Can you work these out from the model? Positions are in its coordinate system, mm. A direction names the side the tool comes from. Round coordinates to 2 decimals unless told otherwise and drop trailing zeros. Write each loop counter-clockwise with the first axis right and the second up, starting at its lowest first coordinate (ties: lowest second). Pieces come first, ordered by that corner, then holes. Notation, with made-up numbers: M 18,1 L 74,1 A29 cw 74,22 Z; hole C 87.5,-17.75 d3. An arc over 180 degrees is marked long. Answer in a Markdown table with one row per item. Add a question column.
(1) For faces 4 (the face through (48, 3, 2)), 5 (the face through (35.1, 3, -10)), 6 (the face through (81, 3, 2)), 7 (the face through (5, 3, 2)), 8 (the face through (2, 3, -8)), which set-ups out of +Z, -Z, +X, -X, +Y, -Y let a thin tool reach every point of the face, with its end or its side?
(2) Suppose I cut it at C-C, the plane x = 45. Write out the boundary of the cut face in (y, z), then the cut area to 3 significant figures.
(3) Suppose I cut it at B-B, the plane z = -11.5. Write out the boundary of the cut face in (x, y).
(4) If we mould it in two halves opening along X, with no side actions, what happens to faces 1 (the face through (59, 3, 0)), 2 (the face through (78.8, 3, -10)), 3 (the face through (42, 6, -4))? For each: released by +X, released by -X, zero draft, split by the parting line, or undercut.
(5) I'm going to push flat-ended pins straight in: pin 1 (1.5 mm diameter, centred on x = 83.5, y = 2, fed in from +Z); pin 2 (1.8 mm diameter, centred on x = 83.5, y = 4, fed in from -Z); pin 3 (1.5 mm diameter, centred on y = 2, z = -11, fed in from +X). Where does each tip first touch, or does it pass through?
(6) Suppose I cut it at D-D, the plane x = 22. Write out the boundary of the cut face in (y, z), then the cut area to 3 significant figures.
(7) Suppose I cut it at A-A, the plane z = 4.25. Write out the boundary of the cut face in (x, y), then the cut area to 3 significant figures.
(8) If I drill on probe 1 along X at (y, z) = (2.3, 3.75); probe 2 along X at (y, z) = (4.2, -11.5); probe 3 along Z at (x, y) = (80, 4.5), over which ranges is the centre line in solid material (lowest first)?
from build123d import *

# Parameters (mm, degrees)
SKETCH1_W               = 86
SKETCH1_H               = 8
BOSS_EXTRUDE1_DEPTH     = 6
SKETCH234_W             = 10
SKETCH234_H             = 6
BOSS_EXTRUDE234_DEPTH   = 6
FILLET134_R             = 1
SKETCH2341_W            = 10
SKETCH2341_H            = 6
BOSS_EXTRUDE2341_DEPTH  = 6
FILLET1341_R            = 1
SKETCH2342_W            = 10
SKETCH2342_H            = 6
BOSS_EXTRUDE2342_DEPTH  = 6
FILLET1342_R            = 1
SKETCH2343_W            = 10
SKETCH2343_H            = 6
BOSS_EXTRUDE2343_DEPTH  = 6
FILLET1343_R            = 1
SKETCH2348_W            = 6
SKETCH2348_H            = 6
BOSS_EXTRUDE2348_DEPTH  = 6
FILLET1348_R            = 1
SKETCH23410_W           = 6
SKETCH23410_H           = 6
BOSS_EXTRUDE23410_DEPTH = 6
FILLET13410_R           = 1


with BuildPart() as part:
    # Sketch1 → Boss-Extrude1 (new body)
    with BuildSketch(Plane(origin=(0, 0, 0), x_dir=(1, 0, 0), z_dir=(0, 1, 0))):
        with Locations((43, 4)):
            Rectangle(SKETCH1_W, SKETCH1_H)
    extrude(amount=BOSS_EXTRUDE1_DEPTH)

    # Sketch234 → Boss-Extrude234 (add)
    with BuildSketch(Plane(origin=(9.232221392, 0, 0), x_dir=(1, 0, 0), z_dir=(0, 0, 1))):
        with Locations((0.767778608, 3)):
            Rectangle(SKETCH234_W, SKETCH234_H)
    extrude(amount=BOSS_EXTRUDE234_DEPTH)

    # Fillet134
    fillet134_edges = [part.edges().sort_by_distance(p)[0] for p in [
        (5, 3, 6),
        (15, 3, 6),
    ]]
    fillet(fillet134_edges, radius=FILLET134_R)

    # Sketch2341 → Boss-Extrude2341 (add)
    with BuildSketch(Plane(origin=(42.232221392, 0, 0), x_dir=(1, 0, 0), z_dir=(0, 0, 1))):
        with Locations((0.767778608, 3)):
            Rectangle(SKETCH2341_W, SKETCH2341_H)
    extrude(amount=BOSS_EXTRUDE2341_DEPTH)

    # Fillet1341
    fillet1341_edges = [part.edges().sort_by_distance(p)[0] for p in [
        (48, 3, 6),
        (38, 3, 6),
    ]]
    fillet(fillet1341_edges, radius=FILLET1341_R)

    # Sketch2342 → Boss-Extrude2342 (add)
    with BuildSketch(Plane(origin=(75.232221392, 0, 0), x_dir=(1, 0, 0), z_dir=(0, 0, 1))):
        with Locations((0.767778608, 3)):
            Rectangle(SKETCH2342_W, SKETCH2342_H)
    extrude(amount=BOSS_EXTRUDE2342_DEPTH)

    # Fillet1342
    fillet1342_edges = [part.edges().sort_by_distance(p)[0] for p in [
        (81, 3, 6),
        (71, 3, 6),
    ]]
    fillet(fillet1342_edges, radius=FILLET1342_R)

    # Sketch2343 → Boss-Extrude2343 (add)
    with BuildSketch(Plane(origin=(73.032221392, 6, -8), x_dir=(1, 0, 0), z_dir=(0, 0, -1))):
        with Locations((0.767778608, 3)):
            Rectangle(SKETCH2343_W, SKETCH2343_H)
    extrude(amount=BOSS_EXTRUDE2343_DEPTH)

    # Fillet1343
    fillet1343_edges = [part.edges().sort_by_distance(p)[0] for p in [
        (68.8, 3, -14),
        (78.8, 3, -14),
    ]]
    fillet(fillet1343_edges, radius=FILLET1343_R)

    # Sketch2348 → Boss-Extrude2348 (add)
    with BuildSketch(Plane(origin=(31.332221392, 6, -8), x_dir=(1, 0, 0), z_dir=(0, 0, -1))):
        with Locations((0.767778608, 3)):
            Rectangle(SKETCH2348_W, SKETCH2348_H)
    extrude(amount=BOSS_EXTRUDE2348_DEPTH)

    # Fillet1348
    fillet1348_edges = [part.edges().sort_by_distance(p)[0] for p in [
        (35.1, 3, -14),
        (29.1, 3, -14),
    ]]
    fillet(fillet1348_edges, radius=FILLET1348_R)

    # Sketch23410 → Boss-Extrude23410 (add)
    with BuildSketch(Plane(origin=(6.532221392, 6, -8), x_dir=(1, 0, 0), z_dir=(0, 0, -1))):
        with Locations((0.767778608, 3)):
            Rectangle(SKETCH23410_W, SKETCH23410_H)
    extrude(amount=BOSS_EXTRUDE23410_DEPTH)

    # Fillet13410
    fillet13410_edges = [part.edges().sort_by_distance(p)[0] for p in [
        (10.3, 3, -14),
        (4.3, 3, -14),
    ]]
    fillet(fillet13410_edges, radius=FILLET13410_R)


solid = part.part
Calculated:
| question | item | result |
|---|---|---|
| 1 | face 4 | +Z, +Y, -Y |
| 1 | face 5 | -Z, +Y, -Y |
| 1 | face 6 | +Z, +X, +Y, -Y |
| 1 | face 7 | +Z, -X, +Y, -Y |
| 1 | face 8 | -Z, -X, +Y, -Y |
| 2 | outline | M 0,-8 L 6,-8 L 6,6 L 0,6 Z |
| 2 | area | 84.0 mm² |
| 3 | outline | M 4.3,0 L 10.3,0 L 10.3,6 L 4.3,6 Z; M 29.1,0 L 35.1,0 L 35.1,6 L 29.1,6 Z; M 68.8,0 L 78.8,0 L 78.8,6 L 68.8,6 Z |
| 4 | face 1 | undercut |
| 4 | face 2 | released by +X |
| 4 | face 3 | zero draft |
| 5 | pin 1 | z = 0 |
| 5 | pin 2 | z = -8 |
| 5 | pin 3 | x = 78.8 |
| 6 | outline | M 0,-8 L 6,-8 L 6,0 L 0,0 Z |
| 6 | area | 48.0 mm² |
| 7 | outline | M 5,0 L 15,0 L 15,6 L 5,6 Z; M 38,0 L 48,0 L 48,6 L 38,6 Z; M 71,0 L 81,0 L 81,6 L 71,6 Z |
| 7 | area | 180 mm² |
| 8 | probe 1 | 5 to 15, 38 to 48, 71 to 81 |
| 8 | probe 2 | 4.3 to 10.3, 29.1 to 35.1, 68.8 to 78.8 |
| 8 | probe 3 | -8 to 6 |
